Work out the finished part from the listing and answer in its coordinate system (mm). A direction names the side the tool comes from. Give positions to 0.01 mm unless a question says otherwise; leave off trailing zeros. Write each loop counter-clockwise with the first axis right and the second up, starting at its lowest first coordinate (ties: lowest second). Pieces come first, ordered by that corner, then holes. Notation, with made-up numbers: (-15.5, 50) -> (35.5, 50) arc R22 cw to (35.5, 62) -> close; hole circle Ø7 at (13.25, -24). An arc over 180 degrees is marked (long way). Use a Markdown table: item, result. Add a question column.
Q1. Section A-A, the plane x = 0 is taken. Give the vertices of the cut face in (y, z).
Q2. For a pull along X with two mould halves and no side action, classify faces 4 (the face through (0, 1, 2.54)), 5 (the face through (10, 12.7, 2)) as pulls with the +X half, pulls with the -X half, needs draft (parallel to the pull), parting line crosses it, or undercut.
Q3. Section B-B, the plane z = 2.1 is taken. Give the vertices of the cut face in (x, y), plus the area to 3 significant figures.
Q4. For faces 1 (the face through (0, 9, 2.54)), 2 (the face through (5.23, 10.69, 1.25)), 3 (the face through (5.44, 7.84, 1.25)), determine the directions among +Z, -Z, +X, -X, +Y, -Y from which every point of the face is accessible in a straight line to the end or side of a thin tool.
Q5. This flat-tipped pin is pushed along its axis until it touches: pin 1 Ø6.5 at (x, y) = (3, 8.5) entering from +Z. Where does it stop, or does it pass through?
Q6. Consider line 1 (X direction, y = 4.5, z = 0.9); line 2 (Y direction, x = 5.25, z = 2.45); line 3 (Y direction, x = 2.25, z = 0.2). Determine where each line is inside the solid, lowest interval first.
Q7. Section C-C, the plane y = -2 is taken. Give the vertices of the cut face in (x, z).
Q8. Section D-D, the plane y = -8.5 is taken. Give the vertices of the cut face in (x, z), plus the area to 3 significant figures.
from build123d import *

# Parameters (mm, degrees)
F1_DEPTH = 3.048
F3_DEPTH = 2.54
F4_W     = 29.287648
F4_H     = 1.191522
F5_DEPTH = 0.508


with BuildPart() as f1:
    # F0 (on Top) → F1 (new body)
    with BuildSketch(Plane.XY):
        with BuildLine():
            Line((12.7, 0), (12.7, 12.7))
            Line((12.7, 12.7), (7.62, 12.7))
            Line((7.62, 12.7), (7.62, 0))
            ThreePointArc((7.62, 0), (0, -7.62), (-7.62, 0))
            Line((-7.62, 0), (-7.62, 12.7))
            Line((-7.62, 12.7), (-12.7, 12.7))
            Line((-12.7, 12.7), (-12.7, 0))
            ThreePointArc((-12.7, 0), (0, -12.7), (12.7, 0))
        make_face()
    extrude(amount=F1_DEPTH)

    # F2 (on Top) → F3 (join)
    with BuildSketch(Plane.XY):
        Polygon((-4.612858, 9.695881), (-8.65593, 11.129335), (-8.692686, 9.47535), (-4.351111, 6.134733), (-0.97243, 8.36986), (3.321907, 6.452318), (9.611405, 10.578007), (8.770715, 11.859614), (2.770109, 9.877271), (-0.53303, 12.011459), align=None)
        Polygon((-4.860972, 2.074731), (-8.904044, 3.508184), (-8.940799, 1.8542), (-4.599224, -1.486418), (-1.220543, 0.74871), (3.073793, -1.168832), (9.363291, 2.956856), (8.522601, 4.238464), (2.521995, 2.256121), (-0.781144, 4.390309), align=None)
    extrude(amount=F3_DEPTH)

    # F4 (on face) → F5 (cut)
    with BuildSketch(Plane.XY.offset(3.048)):
        Rectangle(F4_W, F4_H)
    extrude(amount=-F5_DEPTH, mode=Mode.SUBTRACT)


solid = f1.part
Result set:
| question | item | result |
|---|---|---|
| 1 | outline | (-12.7, 0) -> (-7.62, 0) -> (-7.62, 3.05) -> (-12.7, 3.05) -> close; (0.2, 0) -> (3.89, 0) -> (3.89, 2.54) -> (0.2, 2.54) -> close; (7.94, 0) -> (11.67, 0) -> (11.67, 2.54) -> (7.94, 2.54) -> close |
| 2 | face 4 | undercut |
| 2 | face 5 | needs draft |
| 3 | outline | (-12.7, 0) arc R12.7 ccw to (12.7, 0) -> (12.7, 12.7) -> (7.62, 12.7) -> (7.62, 11.48) -> (2.77, 9.88) -> (-0.53, 12.01) -> (-4.61, 9.7) -> (-7.62, 10.76) -> (-7.62, 12.7) -> (-12.7, 12.7) -> close; hole (-7.62, 0) arc R7.62 ccw to (7.62, 0) -> (7.62, 1.81) -> (3.07, -1.17) -> (-1.22, 0.75) -> (-4.6, -1.49) -> (-7.62, 0.84) -> close; hole (-7.62, 3.05) -> (-4.86, 2.07) -> (-0.78, 4.39) -> (2.52, 2.26) -> (7.62, 3.94) -> (7.62, 9.27) -> (3.32, 6.45) -> (-0.97, 8.37) -> (-4.35, 6.13) -> (-7.62, 8.65) -> close |
| 3 | area | 389 mm2 |
| 4 | face 1 | +Z, +Y |
| 4 | face 2 | +Z, -Z, +Y |
| 4 | face 3 | +Z, -Z |
| 5 | pin 1 | stops at z = 2.54 |
| 6 | line 1 | x = -12.7 to -7.62, 7.62 to 12.7 |
| 6 | line 2 | y = -11.56 to -5.52, 0.26 to 3.16, 7.72 to 10.7 |
| 6 | line 3 | y = -12.5 to -7.28, -0.8 to 2.43, 6.93 to 10.21 |
| 7 | outline | (-12.54, 0) -> (-7.35, 0) -> (-7.35, 3.05) -> (-12.54, 3.05) -> close; (7.35, 0) -> (12.54, 0) -> (12.54, 3.05) -> (7.35, 3.05) -> close |
| 8 | outline | (-9.44, 0) -> (9.44, 0) -> (9.44, 3.05) -> (-9.44, 3.05) -> close |
| 8 | area | 57.5 mm2 |
